Work out the finished part from the listing and answer in its coordinate system (mm). Face numbers are marked on the shaded views. Coordinates: 2 decimals unless noted, no trailing zeros. Loops run counter-clockwise (first coordinate to the right, second up) from the corner with the lowest first, then second, coordinate; pieces in that order, holes last. Notation, with made-up numbers: (80, 60) -> (129, 60) arc R3 ccw to (129, 64) -> close; hole circle Ø5 at (6.25, -8). An arc over 180 degrees is marked (long way). Use a Markdown table: item, result. Add a question column.
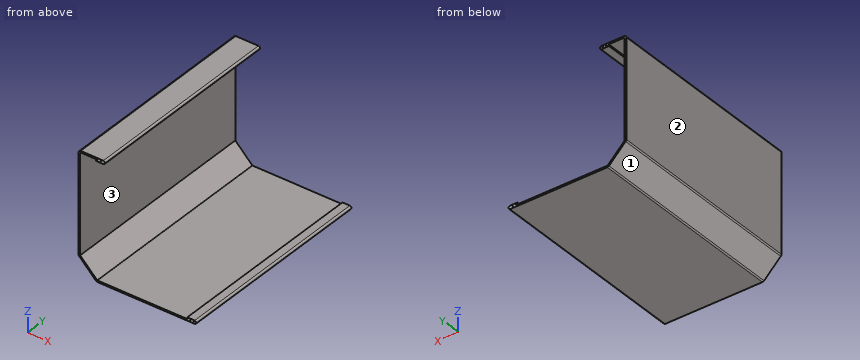
```python
from build123d import *

# Parameters (mm, degrees)
BASE_FLANGE1_DEPTH = 96
HEM1_START         = -96
HEM1_DEPTH         = 192
HEM1_2_DEPTH       = 192


# Read off the part's stored shape, not the designer's step: Hem1
# Sheet-metal steps are written as plain solids
with BuildPart() as part:
    # Sketch1 → Base-Flange1 (new, symmetric)
    with BuildSketch(Plane(origin=(0, 0, 0), x_dir=(-1, 0, 0), z_dir=(0, 1, 0))):
        with BuildLine():
            Line((0, 0), (93.073569946, 0))
            ThreePointArc((93.073569946, 0), (93.929479711, 0.170251038), (94.655084973, 0.655084973))
            Line((94.655084973, 0.655084973), (110.344915027, 16.344915027))
            ThreePointArc((110.344915027, 16.344915027), (110.829748962, 17.070520289), (111, 17.926430054))
            Line((111, 17.926430054), (111, 110.3634))
            ThreePointArc((111, 110.3634), (110.344915027, 111.944915027), (108.7634, 112.6))
            Line((108.7634, 112.6), (86.118343195, 112.6))
            Line((86.118343195, 112.6), (86.118343195, 111.1))
            Line((86.118343195, 111.1), (108.7634, 111.1))
            ThreePointArc((108.7634, 111.1), (109.284254855, 110.884254855), (109.5, 110.3634))
            Line((109.5, 110.3634), (109.5, 17.926430054))
            ThreePointArc((109.5, 17.926430054), (109.443929664, 17.644545437), (109.284254855, 17.405575199))
            Line((109.284254855, 17.405575199), (93.594424801, 1.715745145))
            ThreePointArc((93.594424801, 1.715745145), (93.355454563, 1.556070336), (93.073569946, 1.5))
            Line((93.073569946, 1.5), (0, 1.5))
            Line((0, 1.5), (0, 0))
        make_face()
    extrude(amount=BASE_FLANGE1_DEPTH, both=True)

    # Hem1 outline → Hem1 (cut)
    with BuildSketch(Plane(origin=(0, 0, 0), x_dir=(1, 0, 0), z_dir=(0, 1, 0)).offset(HEM1_START)):
        with BuildLine():
            Line((-86.118343195, -111.1), (-86.119149857, -111.1))
            ThreePointArc((-86.119149857, -111.1), (-86.590150262, -112.163552873), (-87.668343195, -112.6))
            Line((-87.668343195, -112.6), (-86.118343195, -112.6))
            Line((-86.118343195, -112.6), (-86.118343195, -111.1))
        make_face()
        with BuildLine():
            ThreePointArc((-1.55, 0), (-0.471807067, -0.436447127), (-0.000806662, -1.5))
            Line((-0.000806662, -1.5), (0, -1.5))
            Line((0, -1.5), (0, 0))
            Line((0, 0), (-1.55, 0))
        make_face()
    extrude(amount=HEM1_DEPTH, mode=Mode.SUBTRACT)

    # Hem1 2 outline → Hem1 2 (add)
    with BuildSketch(Plane(origin=(0, 0, 0), x_dir=(1, 0, 0), z_dir=(0, 1, 0)).offset(HEM1_START)):
        with BuildLine():
            Line((-94.618343195, -109.5), (-94.618343195, -111))
            Line((-94.618343195, -111), (-87.668343195, -111))
            ThreePointArc((-87.668343195, -111), (-87.618343195, -111.05), (-87.668343195, -111.1))
            Line((-87.668343195, -111.1), (-86.119149857, -111.1))
            ThreePointArc((-86.119149857, -111.1), (-86.554790322, -109.971807067), (-87.668343195, -109.5))
            Line((-87.668343195, -109.5), (-94.618343195, -109.5))
        make_face()
        with BuildLine():
            Line((-8.5, -1.6), (-8.5, -3.1))
            Line((-8.5, -3.1), (-1.55, -3.1))
            ThreePointArc((-1.55, -3.1), (-0.436447127, -2.628192933), (-0.000806662, -1.5))
            Line((-0.000806662, -1.5), (-1.55, -1.5))
            ThreePointArc((-1.55, -1.5), (-1.5, -1.55), (-1.55, -1.6))
            Line((-1.55, -1.6), (-8.5, -1.6))
        make_face()
    extrude(amount=HEM1_2_DEPTH)


solid = part.part
```
Item 1: Section B-B (y = -47) is taken. Determine the outline of the cut face in (x, z).
Item 2: Section D-D (x = -72) is taken. Determine the outline of the cut face in (y, z), then the cut area to 3 significant figures.
Item 3: Section A-A (x = -103.5) is taken. Determine the outline of the cut face in (y, z).
Item 4: Find the intervals of material crossed by probe 1 along Z at (x, y) = (-48, 52); probe 2 along X at (y, z) = (-83.5, 46); probe 3 along Z at (x, y) = (-103.5, 1.5), in increasing order.
Item 5: For a pull along Z with two mould halves and no side action, classify the marked faces 1, 2 and 3 as +Z half, -Z half, draft (parallel to the pull), parting line (faces both ways), or undercut.
Item 6: Section C-C (z = 80) is taken. Determine the outline of the cut face in (x, y).
Item 7: Given pin 1 (7.5 mm diameter, centred on x = -6.5, y = -29.5, fed in from +Z); pin 2 (5 mm diameter, centred on y = 38, z = 83, fed in from +X); pin 3 (17 mm diameter, centred on x = -100, y = 13.5, fed in from -Z), each flat-ended and moving along its own axis, determine where each tip first touches the part or whether it passes through.
Output:
| question | item | result |
|---|---|---|
| 1 | outline | (-111, 17.93) arc R2.24 ccw to (-110.34, 16.34) -> (-94.66, 0.66) arc R2.24 ccw to (-93.07, 0) -> (-1.55, 0) arc R1.55 ccw to (-1.55, 3.1) -> (-8.5, 3.1) -> (-8.5, 1.6) -> (-1.55, 1.6) arc R0.05 cw to (-1.55, 1.5) -> (-93.07, 1.5) arc R0.74 cw to (-93.59, 1.72) -> (-109.28, 17.41) arc R0.74 cw to (-109.5, 17.93) -> (-109.5, 110.36) arc R0.74 cw to (-108.76, 111.1) -> (-87.67, 111.1) arc R0.05 cw to (-87.67, 111) -> (-94.62, 111) -> (-94.62, 109.5) -> (-87.67, 109.5) arc R1.55 ccw to (-87.67, 112.6) -> (-108.76, 112.6) arc R2.24 ccw to (-111, 110.36) -> close |
| 2 | outline | (-96, 0) -> (96, 0) -> (96, 1.5) -> (-96, 1.5) -> close |
| 2 | area | 288 mm2 |
| 3 | outline | (-96, 9.5) -> (96, 9.5) -> (96, 11.62) -> (-96, 11.62) -> close; (-96, 111.1) -> (96, 111.1) -> (96, 112.6) -> (-96, 112.6) -> close |
| 4 | probe 1 | z = 0 to 1.5 |
| 4 | probe 2 | x = -111 to -109.5 |
| 4 | probe 3 | z = 9.5 to 11.62, 111.1 to 112.6 |
| 5 | face 1 | -Z half |
| 5 | face 2 | draft |
| 5 | face 3 | undercut |
| 6 | outline | (-111, -96) -> (-109.5, -96) -> (-109.5, 96) -> (-111, 96) -> close |
| 7 | pin 1 | stops at z = 3.1 |
| 7 | pin 2 | stops at x = -109.5 |
| 7 | pin 3 | stops at z = 0 |
